Geometry: final body of the model. Coordinates: model frame, mm. A direction names the side the tool comes from. Give positions to 0.01 mm unless a question says otherwise; leave off trailing zeros. Loops run counter-clockwise (first coordinate to the right, second up) from the corner with the lowest first, then second, coordinate; pieces in that order, holes last. Notation, with made-up numbers: (-22.75, 72) -> (8.25, 72) arc R4 ccw to (8.25, 77) -> close; hole circle Ø4 at (78.5, 38). An arc over 180 degrees is marked (long way). One line per question, with ' | ' between items. Start each with the question number.
Item 1: Pin query (flat end, axial travel): P1, Ø1, axis at x = 71, y = 213, coming from the +Z side. Return the tip coordinate at first contact, or that it passes through.
Item 2: Mould query, pull axis Y, two halves, no side actions, for faces 1 (the flat face through (0, 197, -162)), 2 (the flat face through (197, 0, -162)), 3 (the flat face through (300, 199, -167)). Classes: released by +Y, released by -Y, zero draft, split by the parting line, or undercut.
Item 3: Section D-D on x = 91. Return loops of the section in (y, z).
Item 4: Section A-A on x = 220.5. Return loops of the section in (y, z), then the cut area to 3 significant figures.
Item 5: Set-up query: faces 4 (the flat face through (350, 198, -15)), 5 (the flat face through (199, 300, -167)), 6 (the flat face through (197, 69, -310)). Return all of +Z, -Z, +X, -X, +Y, -Y with unobstructed straight access to the full face (end or side cutting, diameter ignored); none if empty.
Item 6: Section C-C on z = -69.5. Return loops of the section in (x, y), then the cut area to 3 significant figures.
Item 7: Material intervals for line 1 along Y through (x, z) = (109.5, -173.5); line 2 along Z through (x, y) = (329, 215.5), sorted ascending. Write a range as [from, to].
from build123d import *

# Parameters (mm, degrees)
BOX007_W     = 300
BOX007_H     = 300
BOX007_DEPTH = 10
BOX006_W     = 200
BOX006_H     = 200
BOX006_DEPTH = 300
BOX005_W     = 400
BOX005_H     = 400
BOX005_DEPTH = 300


with BuildPart() as cube006:
    # Box007 → Box007 (new body)
    with BuildSketch(Plane(origin=(50, 50, -20), x_dir=(1, 0, 0), z_dir=(0, 0, 1))):
        with Locations((150, 150)):
            Rectangle(BOX007_W, BOX007_H)
    extrude(amount=BOX007_DEPTH)


with BuildPart() as cube005:
    # Box006 → Box006 (new body)
    with BuildSketch(Plane(origin=(100, 100, -310), x_dir=(1, 0, 0), z_dir=(0, 0, 1))):
        with Locations((100, 100)):
            Rectangle(BOX006_W, BOX006_H)
    extrude(amount=BOX006_DEPTH)


with BuildPart() as cut003:
    # Box005 → Box005 (new body)
    with BuildSketch(Plane.XY.offset(-310)):
        with Locations((200, 200)):
            Rectangle(BOX005_W, BOX005_H)
    extrude(amount=BOX005_DEPTH)

    # Cut002: cut Cube005
    add(cube005.part, mode=Mode.SUBTRACT)

    # Cut003: cut Cube006
    add(cube006.part, mode=Mode.SUBTRACT)


solid = cut003.part
Result sheet:
1) P1: stops at z = -20
2) face 1: zero draft | face 2: released by -Y | face 3: undercut
3) outline: (0, -310) -> (400, -310) -> (400, -10) -> (350, -10) -> (350, -20) -> (50, -20) -> (50, -10) -> (0, -10) -> close
4) outline: (0, -310) -> (100, -310) -> (100, -20) -> (50, -20) -> (50, -10) -> (0, -10) -> close; (300, -310) -> (400, -310) -> (400, -10) -> (350, -10) -> (350, -20) -> (300, -20) -> close | area: 59,000 mm²
5) face 4: +Z | face 5: +Z, -Z | face 6: -Z, +X, -X, +Y, -Y
6) outline: (0, 0) -> (400, 0) -> (400, 400) -> (0, 400) -> close; hole (100, 100) -> (300, 100) -> (300, 300) -> (100, 300) -> close | area: 120,000 mm²
7) line 1: y = [0, 100], [300, 400] | line 2: z = [-310, -20]
